```python
from build123d import *

# Parameters (mm, degrees)
F0_R     = 1.1
F0_R_2   = 1.6
F0_W     = 26
F0_H     = 10
F1_DEPTH = 3.2


with BuildPart() as f1:
    # F0 (on Front) → F1 (new body)
    with BuildSketch(Plane.XZ):
        with BuildLine():
            ThreePointArc((-22, 18), (-16.727922, 5.272078), (-4, 0))
            Line((-4, 0), (4, 0))
            ThreePointArc((4, 0), (16.727922, 5.272078), (22, 18))
            Line((22, 18), (22, 112))
            ThreePointArc((22, 112), (16.727922, 124.727922), (4, 130))
            Line((4, 130), (-4, 130))
            ThreePointArc((-4, 130), (-16.727922, 124.727922), (-22, 112))
            Line((-22, 112), (-22, 18))
        make_face()
        with Locations((-18.274542, 59.802648)):
            Circle(F0_R, mode=Mode.SUBTRACT)
        with Locations((0, 11.6)):
            Circle(F0_R_2, mode=Mode.SUBTRACT)
        Polygon((-5, 25.6), (-13, 25.6), (-13, 67.6), (5, 67.6), (13, 67.6), (13, 25.6), align=None, mode=Mode.SUBTRACT)
        with Locations((0, 79.730161)):
            Circle(F0_R, mode=Mode.SUBTRACT)
        with Locations((0, 98.8)):
            Rectangle(F0_W, F0_H, mode=Mode.SUBTRACT)
        with Locations((1, 118.4)):
            Circle(F0_R_2, mode=Mode.SUBTRACT)
        Polygon((5, 67.6), (-13, 25.6), (-5, 25.6), (13, 67.6), align=None)
    extrude(amount=F1_DEPTH)


solid = f1.part
```
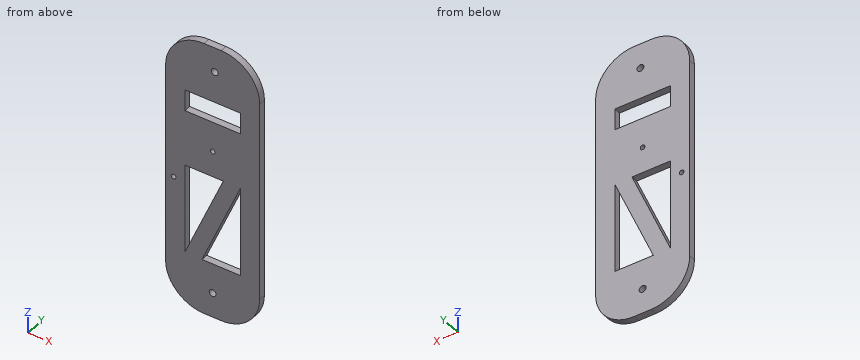
Source: CAD feature listing. Evaluate the final solid. Frame: model axes, mm. Round coordinates to 2 decimals unless told otherwise and drop trailing zeros. Loops run counter-clockwise (first coordinate to the right, second up) from the corner with the lowest first, then second, coordinate; pieces in that order, holes last. Notation, with made-up numbers: M -21.75,-20.5 L -2.75,-20.5 A20 cw -2.75,-12.5 Z; hole C 49,-14 d7. An arc over 180 degrees is marked long. Put each result on its own line as item: value.
(1) Ray query, line 1 (Z direction, x = -9, y = -2.45); line 2 (Z direction, x = 4.5, y = -0.45); line 3 (Z direction, x = -12, y = -0.8). Return the intervals inside material, ascending. Write a range as [from, to].
Solutions:
line 1: [0.71, 34.93], [67.6, 93.8], [103.8, 129.29]
line 2: [0.01, 25.6], [47.77, 66.43], [67.6, 93.8], [103.8, 129.99]
line 3: [1.88, 27.93], [67.6, 93.8], [103.8, 128.12]
(2) Section A-A, the plane z = 118.4. Return loops of the section in (x, y), and give its area (3 significant figures).
Solutions:
outline: M -20.82,-3.2 L -0.6,-3.2 L -0.6,0 L -20.82,0 Z; M 2.6,-3.2 L 20.82,-3.2 L 20.82,0 L 2.6,0 Z
area: 123 mm²
(3) Section C-C, the plane y = -2.6. Return loops of the section in (x, z).
Solutions:
outline: M -22,18 A18 ccw -4,0 L 4,0 A18 ccw 22,18 L 22,112 A18 ccw 4,130 L -4,130 A18 ccw -22,112 Z; hole C -18.27,59.8 d2.2; hole M -13,25.6 L 5,67.6 L -13,67.6 Z; hole M -13,93.8 L 13,93.8 L 13,103.8 L -13,103.8 Z; hole M -5,25.6 L 13,25.6 L 13,67.6 Z; hole C 0,11.6 d3.2; hole C 0,79.73 d2.2; hole C 1,118.4 d3.2
(4) Section B-B, the plane x = 6.5. Return loops of the section in (y, z), and give its area (3 significant figures).
Solutions:
outline: M -3.2,0.17 L 0,0.17 L 0,25.6 L -3.2,25.6 Z; M -3.2,52.43 L 0,52.43 L 0,93.8 L -3.2,93.8 Z; M -3.2,103.8 L 0,103.8 L 0,129.83 L -3.2,129.83 Z
area: 297 mm²
(5) Section D-D, the plane z = 64. Return loops of the section in (x, y), and give its area (3 significant figures).
Solutions:
outline: M -22,-3.2 L -13,-3.2 L -13,0 L -22,0 Z; M 3.46,-3.2 L 11.46,-3.2 L 11.46,0 L 3.46,0 Z; M 13,-3.2 L 22,-3.2 L 22,0 L 13,0 Z
area: 83.2 mm²
(6) First-contact query: pin 1 (1.6 mm diameter, centred on x = -6.5, y = -2, fed in from -Z); pin 2 (4 mm diameter, centred on x = -9.5, z = 65, fed in from +Y). Flat tips, straight axial feed; report the tip coordinate or a pass-through.
Solutions:
pin 1: z = 0.08
pin 2: through
